```python
from build123d import *

# Parameters (mm, degrees)
SKETCH_1_R          = 22.5
EXTRUDE_1_DEPTH     = 10
SKETCH_2_R          = 37.5
EXTRUDE_2_DEPTH     = 10
SKETCH_3_R          = 5
CUT_EXTRUDE_1_DEPTH = 20


with BuildPart() as part:
    # 草图1 → 凸台-拉伸1 (new body)
    with BuildSketch(Plane.XY):
        with Locations((-30.640916886, 5.950554874)):
            Circle(SKETCH_1_R)
    extrude(amount=EXTRUDE_1_DEPTH)

    # 草图2 → 凸台-拉伸2 (add)
    with BuildSketch(Plane.XY.offset(10)):
        with Locations((-30.640916886, 5.950554874)):
            Circle(SKETCH_2_R)
    extrude(amount=EXTRUDE_2_DEPTH)

    # 草图3 → 切除-拉伸1 (cut)
    with BuildSketch(Plane(origin=(0, 0, 0), x_dir=(-1, 0, 0), z_dir=(0, 0, -1))):
        with Locations((30.640916886, 5.950554874)):
            Circle(SKETCH_3_R)
    extrude(amount=-CUT_EXTRUDE_1_DEPTH, mode=Mode.SUBTRACT)


solid = part.part
```
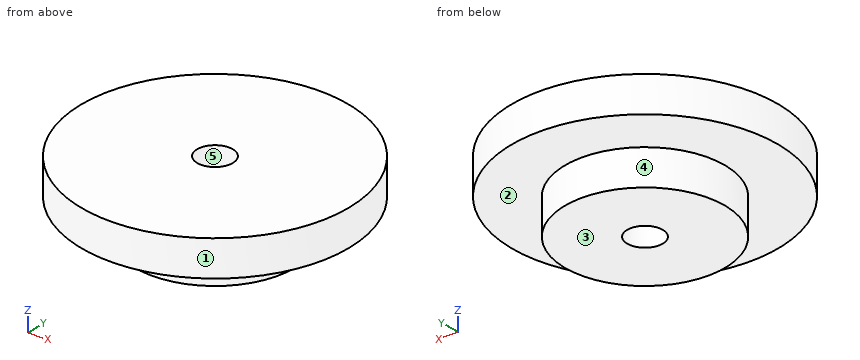
The model under review builds one solid part; all positions refer to its coordinate system, in mm. Face numbers are marked on the shaded views. A direction names the side the tool comes from. Round coordinates to 2 decimals unless told otherwise and drop trailing zeros. Order: outer loops, then holes, each group sorted by start corner. A loop starts at its lowest first (then second) coordinate and runs counter-clockwise, first axis right, second up. Notation, with made-up numbers: (-27.75, 81.25) -> (-16.75, 81.25) arc R33 cw to (-16.75, 109.25) -> close; hole circle Ø4 at (64.5, 65). An arc over 180 degrees is marked (long way). Use a Markdown table: item, result.
Q1. Clearance check with flat-ended pins moving along their axes: P1, Ø2, axis at x = -31, y = 11, coming from the -Z side; P2, Ø2, axis at x = -33, z = 7, coming from the -Y side; P3, Ø6, axis at y = 21, z = 14, coming from the +X side; P4, Ø2, axis at x = -30.5, z = 17.5, coming from the +Y side. State where each tip first meets the part, or that it passes through.
Values:
| item | result |
|---|---|
| P1 | stops at z = 0 |
| P2 | stops at y = -16.51 |
| P3 | stops at x = 4.87 |
| P4 | stops at y = 43.45 |
Q2. We need section A-A on x = -30. Write out the cut boundary in (y, z), then the cut area to 3 significant figures.
Values:
| item | result |
|---|---|
| outline | (-31.54, 10) -> (-16.54, 10) -> (-16.54, 0) -> (0.99, 0) -> (0.99, 20) -> (-31.54, 20) -> close; (10.91, 0) -> (28.44, 0) -> (28.44, 10) -> (43.45, 10) -> (43.45, 20) -> (10.91, 20) -> close |
| area | 1,000 mm^2 |
Q3. Tool access review of the marked faces 1 and 2: name each direction out of +Z, -Z, +X, -X, +Y, -Y from which nothing blocks a thin tool from reaching the whole face with its end or side.
Values:
| item | result |
|---|---|
| face 1 | +Z, -Z |
| face 2 | -Z |
Q4. For line 1 (Z direction, x = -60, y = -10); line 2 (X direction, y = 2, z = 5.5); line 3 (X direction, y = 7.5, z = 8.25), list the stretches that pass through material, from the lowest coordinate up.
Values:
| item | result |
|---|---|
| line 1 | z = 10 to 20 |
| line 2 | x = -52.79 to -33.71, -27.58 to -8.49 |
| line 3 | x = -53.09 to -35.39, -25.89 to -8.19 |
Q5. Mouldability with a two-part tool opening along X and no side actions: class the marked faces 3, 4 and 5 as +X half, -X half, draft (parallel to the pull), parting line (faces both ways), or undercut.
Values:
| item | result |
|---|---|
| face 3 | draft |
| face 4 | parting line |
| face 5 | undercut |
Q6. We need section B-B on y = 2. Write out the cut boundary in (x, z).
Values:
| item | result |
|---|---|
| outline | (-67.93, 10) -> (-52.79, 10) -> (-52.79, 0) -> (-33.71, 0) -> (-33.71, 20) -> (-67.93, 20) -> close; (-27.58, 0) -> (-8.49, 0) -> (-8.49, 10) -> (6.65, 10) -> (6.65, 20) -> (-27.58, 20) -> close |
Q7. We need section C-C on x = -48.5. Write out the cut boundary in (y, z).
Values:
| item | result |
|---|---|
| outline | (-27.02, 10) -> (-7.74, 10) -> (-7.74, 0) -> (19.64, 0) -> (19.64, 10) -> (38.92, 10) -> (38.92, 20) -> (-27.02, 20) -> close |
Q8. We need section D-D on y = 13.5. Write out the cut boundary in (x, z).
Values:
| item | result |
|---|---|
| outline | (-67.37, 10) -> (-51.84, 10) -> (-51.84, 0) -> (-9.45, 0) -> (-9.45, 10) -> (6.09, 10) -> (6.09, 20) -> (-67.37, 20) -> close |
